Autodesk Inventor part; units mm, degrees
ref_plane "YZ Plane" through (0, 0, 0) normal (1, 0, 0) x (0, 1, 0)
ref_plane "XZ Plane" through (0, 0, 0) normal (0, 1, 0) x (-1, 0, 0)
ref_plane "XY Plane" through (0, 0, 0) normal (0, 0, 1) x (1, 0, 0)
sketch "Szkic1" plane through (0, 0, 0) normal (0, 0, 1) x (1, 0, 0)
  arc A0 (0, 35) -> (0, -35) centre (0, 0) ccw
  line L0 (0, 35) -> (390, 35)
  arc A1 (390, -35) -> (390, 35) centre (390, 0) ccw
  line L1 (0, -35) -> (390, -35)
  line L2 (390, 40) -> (0, 40)
  arc A2 (0, 40) -> (0, -40) centre (0, 0) ccw
  line L3 (0, -40) -> (390, -40)
  arc A3 (390, -40) -> (390, 40) centre (390, 0) ccw
  point P0 (424.991, -0.7958)
  dimension "d0" = 70
  dimension "d1" = 390
  dimension "d2" = 70
  dimension "d3" = 5
extrude "Wyciągnięcie proste1" add sketch "Szkic1" along normal blind 120
fillet "Zaokrąglenie1" radius 2 4 edges at (-40, 0, 120) (195, -40, 120) (430, 0, 120) (195, 40, 120)
fillet "Zaokrąglenie2" radius 2 4 edges at (195, 35, 120) (425, 0, 120) (195, -35, 120) (-35, 0, 120)
fillet "Zaokrąglenie3" radius 2 4 edges at (-40, 0, 0) (195, -40, 0) (430, 0, 0) (195, 40, 0)
fillet "Zaokrąglenie4" radius 2 4 edges at (425, 0, 0) (195, -35, 0) (-35, 0, 0) (195, 35, 0)
properties part number "pastran"
For this review, take the finished solid that the model builds, in its own axes (mm). A direction names the side the tool comes from. Round coordinates to 2 decimals unless told otherwise and drop trailing zeros. Order: outer loops, then holes, each group sorted by start corner. A loop starts at its lowest first (then second) coordinate and runs counter-clockwise, first axis right, second up. Notation, with made-up numbers: M -11,7.5 L 1,7.5 A7 ccw 1,20.5 Z; hole C 26,-13 d6. An arc over 180 degrees is marked long. Use a Markdown table: item, result. Add a question column.
Item 1: Insertion check: pin 1 (2 mm diameter, centred on y = -13.5, z = 24.5, fed in from -X); pin 2 (5 mm diameter, centred on y = -29, z = 19, fed in from +X); pin 3 (12 mm diameter, centred on y = -14.5, z = 83.5, fed in from +X). Each pin has a flat end and moves straight along its axis. Give the tip position at first contact, or say it passes through.
Item 2: Add section C-C, the plane x = 276.5. Give the boundary of the cut face in (y, z).
Item 3: Add section A-A, the plane z = 27. Give the boundary of the cut face in (x, y), then the cut area to 3 significant figures.
Item 4: To check wall thickness, follow line 1 along Y through (x, z) = (65, 87.5); line 2 along X through (y, z) = (0.5, 99); line 3 along X through (y, z) = (-18.5, 13.5). State the ranges of each line that lie inside material, in increasing order.
Item 5: Mouldability with a two-part tool opening along Y and no side actions: class faces 1 (the flat face through (198, 40, 59)), 2 (the flat face through (192, -35, 59)), 3 (the flat face through (192, -40, 59)) as released by +Y, released by -Y, zero draft, split by the parting line, or undercut.
Item 6: Add section B-B, the plane y = 0. Give the boundary of the cut face in (x, z), then the cut area to 3 significant figures.
Item 7: Tool access review of faces 4 (the cylindrical face through (-39.99, -0.88, 59.19)), 5 (the cylindrical face through (424.99, 0.77, 59.19)): name each direction out of +Z, -Z, +X, -X, +Y, -Y from which nothing blocks a thin tool from reaching the whole face with its end or side.
Geometry results:
| question | item | result |
|---|---|---|
| 1 | pin 1 | stops at x = -38 |
| 1 | pin 2 | stops at x = 419.96 |
| 1 | pin 3 | stops at x = 429.09 |
| 2 | outline | M -40,2 A2 ccw -38,0 L -37,0 A2 ccw -35,2 L -35,118 A2 ccw -37,120 L -38,120 A2 ccw -40,118 Z; M 35,2 A2 ccw 37,0 L 38,0 A2 ccw 40,2 L 40,118 A2 ccw 38,120 L 37,120 A2 ccw 35,118 Z |
| 3 | outline | M 0,-40 L 390,-40 A40 ccw 390,40 L 0,40 A40 ccw Z; hole M 0,-35 L 390,-35 A35 ccw 390,35 L 0,35 A35 ccw Z |
| 3 | area | 5,080 mm² |
| 4 | line 1 | y = -40 to -35, 35 to 40 |
| 4 | line 2 | x = -40 to -35, 425 to 430 |
| 4 | line 3 | x = -35.46 to -29.71, 419.71 to 425.46 |
| 5 | face 1 | released by +Y |
| 5 | face 2 | undercut |
| 5 | face 3 | released by -Y |
| 6 | outline | M -40,2 A2 ccw -38,0 L -37,0 A2 ccw -35,2 L -35,118 A2 ccw -37,120 L -38,120 A2 ccw -40,118 Z; M 425,2 A2 ccw 427,0 L 428,0 A2 ccw 430,2 L 430,118 A2 ccw 428,120 L 427,120 A2 ccw 425,118 Z |
| 6 | area | 1,190 mm² |
| 7 | face 4 | +Z, -Z, -X |
| 7 | face 5 | +Z, -Z |
